Source: CAD feature listing. Evaluate the final solid. Frame: model axes, mm. A direction names the side the tool comes from. Give positions to 0.01 mm unless a question says otherwise; leave off trailing zeros. Loops run counter-clockwise (first coordinate to the right, second up) from the corner with the lowest first, then second, coordinate; pieces in that order, holes last. Notation, with made-up numbers: M 64.5,7.5 L 105.5,7.5 A15 ccw 105.5,32.5 Z; hole C -20,-0.5 d4. An arc over 180 degrees is marked long. Answer in a Markdown table with one row per item.
```python
from build123d import *

# Parameters (mm, degrees)
F0_R     = 40
F1_DEPTH = 3
F2_DEPTH = 1
F3_R     = 25
F4_DEPTH = 3
F5_T     = -2.5


with BuildPart() as f1:
    # F0 (on Front) → F1 (new body)
    with BuildSketch(Plane.XZ):
        Circle(F0_R)
    extrude(amount=F1_DEPTH)

    # F2 (add): a face of the model
    f2_faces = [f1.faces().sort_by_distance(p)[0] for p in [
        (0, -3, 0),
    ]]
    extrude(f2_faces, amount=F2_DEPTH)

    # F3 (on face) → F4 (join)
    with BuildSketch(Plane(origin=(0, 0, 0), x_dir=(-1, 0, 0), z_dir=(0, 1, 0))):
        Circle(F3_R)
    extrude(amount=F4_DEPTH)

    # F5
    f5_openings = [f1.faces().sort_by_distance(p)[0] for p in [
        (0, -4, 0),
    ]]
    offset(amount=F5_T, openings=f5_openings, kind=Kind.INTERSECTION)


solid = f1.part
```
1) Section A-A, the plane x = 0. Return loops of the section in (y, z), then the cut area to 4 significant figures.
Reply:
| item | result |
|---|---|
| outline | M -4,-40 L 0,-40 L 0,-25 L 3,-25 L 3,25 L 0,25 L 0,40 L -4,40 L -4,37.5 L -2.5,37.5 L -2.5,22.5 L 0.5,22.5 L 0.5,-22.5 L -2.5,-22.5 L -2.5,-37.5 L -4,-37.5 Z |
| area | 222.5 mm² |
2) Section C-C, the plane y = -1.5. Return loops of the section in (x, z).
Reply:
| item | result |
|---|---|
| outline | C 0,0 d80; hole C 0,0 d45 |
3) Section B-B, the plane z = 0. Return loops of the section in (x, y).
Reply:
| item | result |
|---|---|
| outline | M -40,-4 L -37.5,-4 L -37.5,-2.5 L -22.5,-2.5 L -22.5,0.5 L 22.5,0.5 L 22.5,-2.5 L 37.5,-2.5 L 37.5,-4 L 40,-4 L 40,0 L 25,0 L 25,3 L -25,3 L -25,0 L -40,0 Z |
4) Pin query (flat end, axial travel): pin 1 Ø10 at (x, z) = (-29, -13) entering from -Y; pin 2 Ø1 at (x, y) = (7, -0.5) entering from -Z; pin 3 Ø1.5 at (x, y) = (-10.5, 1) entering from +Z. Return the tip coordinate at first contact, or that it passes through.
Reply:
| item | result |
|---|---|
| pin 1 | stops at y = -2.5 |
| pin 2 | stops at z = -39.47 |
| pin 3 | stops at z = 23.02 |
5) Material intervals for L1, parallel to Z at x = 0, y = -1.2; L2, parallel to Z at x = 0, y = -3.55; L3, parallel to Y at x = -22, z = -26.5, sorted ascending.
Reply:
| item | result |
|---|---|
| L1 | z = -40 to -22.5, 22.5 to 40 |
| L2 | z = -40 to -37.5, 37.5 to 40 |
| L3 | y = -2.5 to 0 |
6) Section D-D, the plane x = -33. Return loops of the section in (y, z), then the cut area to 3 significant figures.
Reply:
| item | result |
|---|---|
| outline | M -4,-22.61 L 0,-22.61 L 0,22.61 L -4,22.61 L -4,17.81 L -2.5,17.81 L -2.5,-17.81 L -4,-17.81 Z |
| area | 127 mm² |
7) Pull-direction query (X, two-part tool) for faces 1 (the flat face through (12, -4, 36)), 2 (the cylindrical face through (-10.382, -1.021, -19.961)), 3 (the cylindrical face through (-8.67, -1.97, -39.05)); classes: released by +X, released by -X, zero draft, split by the parting line, or undercut.
Reply:
| item | result |
|---|---|
| face 1 | zero draft |
| face 2 | undercut |
| face 3 | split by the parting line |
8) Set-up query: faces 4 (the flat face through (0, 3, 0)), 5 (the cylindrical face through (-23.846, 1.479, 7.509)), 6 (the flat face through (16.1, -2.5, -16.1)). Return all of +Z, -Z, +X, -X, +Y, -Y with unobstructed straight access to the full face (end or side cutting, diameter ignored); none if empty.
Reply:
| item | result |
|---|---|
| face 4 | +Z, -Z, +X, -X, +Y |
| face 5 | +Y |
| face 6 | -Y |
